The figure shows three views and two pictorial views of one solid part (mm, origin at its lowest corner). Answer the questions. Round coordinates to 2 decimals unless told otherwise and drop trailing zeros. Order: outer loops, then holes, each group sorted by start corner. A loop starts at its lowest first (then second) coordinate and runs counter-clockwise, first axis right, second up. Notation, with made-up numbers: (86, 46.5) -> (106, 46.5) arc R19 cw to (106, 83.5) -> close; hole circle Ø4 at (32, 89.5). An arc over 180 degrees is marked (long way). Return JSON: item names as keys, results as strings. Group by question number.
(1) The part is cut by section B-B (y = 4.75). Determine the outline of the cut face in (x, z).
(2) The part is cut by section A-A (z = 0.85). Determine the outline of the cut face in (x, y).
(3) Consider line 1 (X direction, y = 14.5, z = 0.45); line 2 (Y direction, x = 16.5, z = 1.6); line 3 (X direction, y = 18.25, z = 0.45). Determine where each line is inside the solid, lowest interval first. Write a range as [from, to].
(4) The part is cut by section C-C (x = 98). Determine the outline of the cut face in (y, z).
(5) Each of these flat-tipped pins is pushed along its axis until it touches: pin 1 (1.5 mm diameter, centred on y = 15.5, z = 2, fed in from -X); pin 2 (0.9 mm diameter, centred on x = 14.5, z = 1.5, fed in from +Y); pin 3 (0.9 mm diameter, centred on y = 2.5, z = 2, fed in from +X). Where does it stop, or does it pass through?
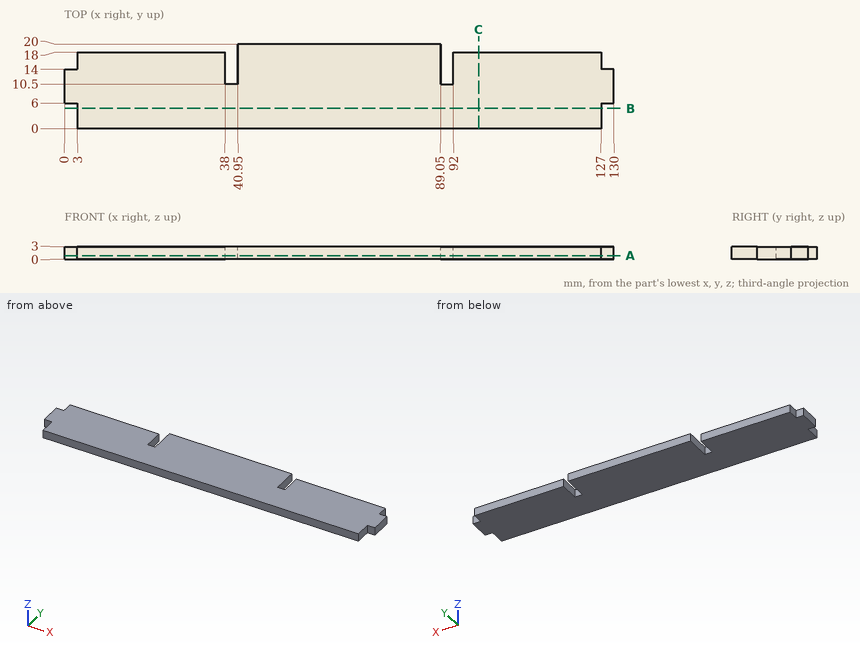
Answer below:
{
 "1": {"outline": "(3, 0) -> (127, 0) -> (127, 3) -> (3, 3) -> close"},
 "2": {"outline": "(0, 6) -> (3, 6) -> (3, 0) -> (127, 0) -> (127, 6) -> (130, 6) -> (130, 14) -> (127, 14) -> (127, 18) -> (92, 18) -> (92, 10.5) -> (89.05, 10.5) -> (89.05, 20) -> (40.95, 20) -> (40.95, 10.5) -> (38, 10.5) -> (38, 18) -> (3, 18) -> (3, 14) -> (0, 14) -> close"},
 "3": {"line 1": "x = [3, 38], [40.95, 89.05], [92, 127]", "line 2": "y = [0, 18]", "line 3": "x = [40.95, 89.05]"},
 "4": {"outline": "(0, 0) -> (18, 0) -> (18, 3) -> (0, 3) -> close"},
 "5": {"pin 1": "stops at x = 3", "pin 2": "stops at y = 18", "pin 3": "stops at x = 127"}
}
